For this review, take the finished solid that the model builds, in its own axes (mm). Coordinates: 2 decimals unless noted, no trailing zeros. Write each loop counter-clockwise with the first axis right and the second up, starting at its lowest first coordinate (ties: lowest second). Pieces come first, ordered by that corner, then holes. Notation, with made-up numbers: M -28,23 L -14,23 A24 ccw -14,36 Z; hole C 62,81 d6. An arc over 180 degrees is marked long. Return JSON: item names as keys, results as strings.
```python
from build123d import *

# Parameters (mm, degrees)
CYLINDER_R        = 1.5
CYLINDER_DEPTH    = 4
CYLINDER002_R     = 3
CYLINDER002_DEPTH = 4
CYLINDER001_R     = 1.5
CYLINDER001_DEPTH = 4
BOX001_W          = 140
BOX001_H          = 20
BOX001_DEPTH      = 4
BOX002_W          = 140
BOX002_H          = 20
BOX002_DEPTH      = 4
BOX_W             = 140
BOX_H             = 4
BOX_DEPTH         = 20


with BuildPart() as obj1:
    # Cylinder → Cylinder (new body)
    with BuildSketch(Plane(origin=(33, 12, 0), x_dir=(1, 0, 0), z_dir=(0, 0, 1))):
        Circle(CYLINDER_R)
    extrude(amount=CYLINDER_DEPTH)


with BuildPart() as cylinder002:
    # Cylinder002 → Cylinder002 (new body)
    with BuildSketch(Plane(origin=(70, -8, 16), x_dir=(1, 0, 0), z_dir=(0, 0, 1))):
        Circle(CYLINDER002_R)
    extrude(amount=CYLINDER002_DEPTH)


with BuildPart() as obj2:
    # Cylinder001 → Cylinder001 (new body)
    with BuildSketch(Plane(origin=(107, 12, 0), x_dir=(1, 0, 0), z_dir=(0, 0, 1))):
        Circle(CYLINDER001_R)
    extrude(amount=CYLINDER001_DEPTH)

    # Fusion001: union obj1, Cylinder002
    add(obj1.part)
    add(cylinder002.part)


with BuildPart() as obj3:
    # Box001 → Box001 (new body)
    with BuildSketch(Plane.XY):
        with Locations((70, 10)):
            Rectangle(BOX001_W, BOX001_H)
    extrude(amount=BOX001_DEPTH)


with BuildPart() as obj4:
    # Box002 → Box002 (new body)
    with BuildSketch(Plane(origin=(0, -16, 16), x_dir=(1, 0, 0), z_dir=(0, 0, 1))):
        with Locations((70, 10)):
            Rectangle(BOX002_W, BOX002_H)
    extrude(amount=BOX002_DEPTH)


with BuildPart() as obj5:
    # Box → Box (new body)
    with BuildSketch(Plane.XY):
        with Locations((70, 2)):
            Rectangle(BOX_W, BOX_H)
    extrude(amount=BOX_DEPTH)

    # Fusion: union obj3, obj4
    add(obj3.part)
    add(obj4.part)

    # Cut: cut obj2
    add(obj2.part, mode=Mode.SUBTRACT)


solid = obj5.part
```
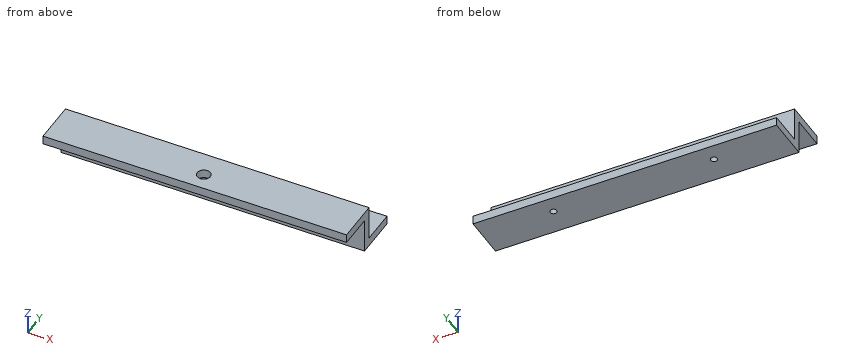
1. Clearance check with flat-ended pins moving along their axes: pin 1 Ø10 at (x, y) = (83.5, -5.5) entering from -Z; pin 2 Ø8 at (x, z) = (60, 11) entering from -Y; pin 3 Ø3.5 at (x, y) = (70, -8) entering from +Z; pin 4 Ø4 at (x, y) = (33, 12) entering from +Z. State where each tip first meets the part, or that it passes through.
Checks:
{"pin 1": "z = 16", "pin 2": "y = 0", "pin 3": "through", "pin 4": "z = 4"}
2. We need section C-C (y = -8). State the section outline as (x, z) points.
Checks:
{"outline": "M 0,16 L 67,16 L 67,20 L 0,20 Z; M 73,16 L 140,16 L 140,20 L 73,20 Z"}
3. Wall thickness on L1, parallel to Y at x = 33, z = 3.15; L2, parallel to X at y = 13, z = 1; L3, parallel to Z at x = 83, y = 11: over which ranges is each line inside the solid? List them lowest first. Write a range as from..to.
Checks:
{"L1": "0..10.5, 13.5..20", "L2": "0..31.88, 34.12..105.88, 108.12..140", "L3": "0..4"}
4. We need section D-D (x = 112.5). State the section outline as (y, z) points, plus the area to 3 significant figures.
Checks:
{"outline": "M -16,16 L 0,16 L 0,0 L 20,0 L 20,4 L 4,4 L 4,20 L -16,20 Z", "area": "208 mm2"}
5. We need section A-A (y = 12). State the section outline as (x, z) points, plus the area to 3 significant figures.
Checks:
{"outline": "M 0,0 L 31.5,0 L 31.5,4 L 0,4 Z; M 34.5,0 L 105.5,0 L 105.5,4 L 34.5,4 Z; M 108.5,0 L 140,0 L 140,4 L 108.5,4 Z", "area": "536 mm2"}
6. We need section B-B (x = 70). State the section outline as (y, z) points, plus the area to 3 significant figures.
Checks:
{"outline": "M -16,16 L -11,16 L -11,20 L -16,20 Z; M -5,16 L 0,16 L 0,0 L 20,0 L 20,4 L 4,4 L 4,20 L -5,20 Z", "area": "184 mm2"}
